Verification items for the finished model (mm, model axes). Round coordinates to 2 decimals unless told otherwise and drop trailing zeros. Loops run counter-clockwise (first coordinate to the right, second up) from the corner with the lowest first, then second, coordinate; pieces in that order, holes last. Notation, with made-up numbers: (44, 87.5) - (54, 87.5) arc R14 ccw to (54, 93.5) - close; hole circle Ø9 at (48, 9.25). An arc over 180 degrees is marked (long way). Use a Markdown table: item, result. Add a question column.
```python
from build123d import *

# Parameters (mm, degrees)
TORUS020_R              = 3.05
CONE003_PITCH_ANGLE     = 90
CYLINDER801_R           = 3.6
CYLINDER801_DEPTH       = 3
CYLINDER801_PITCH_ANGLE = 90
BOX179_W                = 16
BOX179_H                = 10
BOX179_DEPTH            = 10


with BuildPart() as torus:
    # Torus020 → Torus020 (revolve)
    with BuildSketch(Plane(origin=(0, 0, 1), x_dir=(1, 0, 0), z_dir=(0, -1, 0))):
        with Locations((35, 0)):
            Circle(TORUS020_R)
    revolve(axis=Axis((0, 0, 1), (0, 0, 1)))


with BuildPart() as cone:
    # Cone003 → Cone003 (revolve)
    with BuildSketch(Plane.XZ):
        Polygon((0, 0), (2.9, 0), (3.6, 5), (0, 5), align=None)
    revolve(axis=Axis((0, 0, 0), (0, 0, 1)))


with BuildPart() as cone_1:
    # Cone003 pitch: moved
    add(cone.part.rotate(Axis((0, 0, 0), (0, 1, 0)), CONE003_PITCH_ANGLE))


with BuildPart() as cone_2:
    # Cone003 placement: moved
    add(cone_1.part.moved(Location((34.95, 0, 0))))


with BuildPart() as cut:
    # Cylinder801 → Cylinder801 (new body)
    with BuildSketch(Plane.XY):
        Circle(CYLINDER801_R)
    extrude(amount=CYLINDER801_DEPTH)


with BuildPart() as cut_1:
    # Cylinder801 pitch: moved
    add(cut.part.rotate(Axis((0, 0, 0), (0, 1, 0)), CYLINDER801_PITCH_ANGLE))


with BuildPart() as cut_2:
    # Cylinder801 placement: moved
    add(cut_1.part.moved(Location((39.95, 0, 0))))

    # Fusion611: union Cone
    add(cone_2.part)


with BuildPart() as cut_3:
    # Fusion611 placement: moved
    add(cut_2.part.moved(Location((1, 0, 1))))

    # Cut066379: cut Torus
    add(torus.part, mode=Mode.SUBTRACT)


with BuildPart() as obj1:
    # Box179 → Box179 (new body)
    with BuildSketch(Plane(origin=(37, -5, -3), x_dir=(1, 0, 0), z_dir=(0, 0, 1))):
        with Locations((8, 5)):
            Rectangle(BOX179_W, BOX179_H)
    extrude(amount=BOX179_DEPTH)

    # Common053: intersect Cut
    add(cut_3.part, mode=Mode.INTERSECT)


with BuildPart() as obj1_1:
    # Common053 placement: moved
    add(obj1.part.moved(Location((0, 0, -1))))


solid = obj1_1.part
```
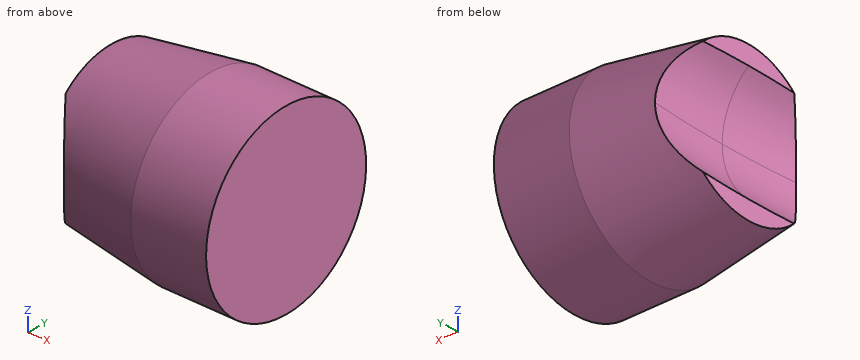
Q1. Go/stop test with flat-tipped pins: pin 1 Ø4 at (x, z) = (39.5, 1.5) entering from -Y; pin 2 Ø2 at (x, z) = (38.5, -1.5) entering from -Y. Record where each tip stops, or that it passes through.
Q2. Section check B-B on x = 38.75. Record the cut outline in (y, z).
Q3. Section check A-A on x = 43. Record the cut outline in (y, z), plus the area to 3 significant figures.
Q4. Thickness scan on line 1 along Z through (x, y) = (37.5, 0.75); line 2 along X through (y, z) = (0, -1.25); line 3 along Y through (x, z) = (39, 1.75). Record the ranges inside material, lowest first.
Determined:
| question | item | result |
|---|---|---|
| 1 | pin 1 | stops at y = -3.6 |
| 1 | pin 2 | stops at y = -3.27 |
| 2 | outline | circle Ø6.58 at (0, 0) |
| 3 | outline | circle Ø7.2 at (0, 0) |
| 3 | area | 40.7 mm² |
| 4 | line 1 | z = -3.03 to -1.74, 1.74 to 3.03 |
| 4 | line 2 | x = 37.78 to 43.95 |
| 4 | line 3 | y = -2.83 to 2.83 |
